For this review, take the finished solid that the model builds, in its own axes (mm). A direction names the side the tool comes from. Round coordinates to 2 decimals unless told otherwise and drop trailing zeros. Write each loop counter-clockwise with the first axis right and the second up, starting at its lowest first coordinate (ties: lowest second). Pieces come first, ordered by that corner, then holes. Notation, with made-up numbers: M -10.5,-6 L 12.5,-6 A17 ccw 12.5,19 Z; hole C 45,39 d1. An arc over 180 degrees is marked long. Answer in a Markdown table with one row per item.
```python
from build123d import *

# Parameters (mm, degrees)
SKETCH1_W               = 195
SKETCH1_H               = 20
BOSS_EXTRUDE1_DEPTH     = 4.9
SKETCH2_R               = 1.75
CUT_EXTRUDE1_DEPTH      = 6
CUT_EXTRUDE2_START      = -2
CUT_EXTRUDE2_DEPTH      = 4.25
SKETCH4_W               = 5.75
SKETCH4_H               = 4.25
CUT_EXTRUDE3_DEPTH      = 5.9
LPATTERN1_COUNT         = 3
LPATTERN1_PITCH         = 35
MIRROR1_COPY_1_SKETCH_R = 1.75
MIRROR1_COPY_1_DEPTH    = 6
MIRROR1_COPY_2_SKETCH_R = 1.75
MIRROR1_COPY_2_DEPTH    = 6
MIRROR1_START           = -2
MIRROR1_COPY_3_DEPTH    = 4.25
MIRROR1_COPY_4_DEPTH    = 4.25
MIRROR1_COPY_5_SKETCH_W = 5.75
MIRROR1_COPY_5_SKETCH_H = 4.25
MIRROR1_COPY_5_DEPTH    = 5.9
MIRROR1_COPY_6_SKETCH_W = 5.75
MIRROR1_COPY_6_SKETCH_H = 4.25
MIRROR1_COPY_6_DEPTH    = 5.9
SKETCH5_R               = 4.25
CUT_EXTRUDE4_DEPTH      = 6
CUT_EXTRUDE5_START      = -4.8
SKETCH6_R               = 2.625
CUT_EXTRUDE5_DEPTH      = 11.8
LPATTERN2_COUNT         = 2
LPATTERN2_PITCH         = 35
MIRROR2_COPY_1_SKETCH_R = 4.25
MIRROR2_COPY_1_DEPTH    = 6
MIRROR2_START           = -4.8
MIRROR2_COPY_2_SKETCH_R = 2.625
MIRROR2_COPY_2_DEPTH    = 11.8


with BuildPart() as part:
    # Sketch1 → Boss-Extrude1 (new body, symmetric)
    with BuildSketch(Plane.XY):
        Rectangle(SKETCH1_W, SKETCH1_H)
    extrude(amount=BOSS_EXTRUDE1_DEPTH, both=True)

    # Sketch2 → Cut-Extrude1 (cut)
    with BuildSketch(Plane(origin=(0, 10, 0), x_dir=(1, 0, 0), z_dir=(0, 1, 0))):
        with Locations((-87.5, 0)):
            Circle(SKETCH2_R)
    cut_extrude1 = extrude(amount=-CUT_EXTRUDE1_DEPTH, mode=Mode.SUBTRACT)

    # Sketch3 → Cut-Extrude2 (cut)
    with BuildSketch(Plane(origin=(0, 10, 0), x_dir=(1, 0, 0), z_dir=(0, 1, 0)).offset(CUT_EXTRUDE2_START)):
        Polygon((-87.5, 3.319764048), (-90.375, 1.659882024), (-90.375, -1.659882024), (-87.5, -3.319764048), (-84.625, -1.659882024), (-84.625, 1.659882024), align=None)
    cut_extrude2 = extrude(amount=-CUT_EXTRUDE2_DEPTH, mode=Mode.SUBTRACT)

    # Sketch4 → Cut-Extrude3 (cut, through all)
    with BuildSketch(Plane.XY):
        with Locations((-87.5, 5.875)):
            Rectangle(SKETCH4_W, SKETCH4_H)
    cut_extrude3 = extrude(amount=CUT_EXTRUDE3_DEPTH, mode=Mode.SUBTRACT)

    # LPattern1: Cut-Extrude1, Cut-Extrude2, Cut-Extrude3 ×3
    with Locations(*[(i * LPATTERN1_PITCH, 0, 0) for i in range(1, LPATTERN1_COUNT)]):
        add(cut_extrude1, mode=Mode.SUBTRACT)
        add(cut_extrude2, mode=Mode.SUBTRACT)
        add(cut_extrude3, mode=Mode.SUBTRACT)

    # Mirror1: Cut-Extrude1, Cut-Extrude2, Cut-Extrude3 across plane
    add(cut_extrude1.mirror(Plane(origin=(0, 0, 0), x_dir=(0, 0, 1), z_dir=(1, 0, 0))), mode=Mode.SUBTRACT)
    add(cut_extrude2.mirror(Plane(origin=(0, 0, 0), x_dir=(0, 0, 1), z_dir=(1, 0, 0))), mode=Mode.SUBTRACT)
    add(cut_extrude3.mirror(Plane(origin=(0, 0, 0), x_dir=(0, 0, 1), z_dir=(1, 0, 0))), mode=Mode.SUBTRACT)

    # Mirror1 copy 1 sketch → Mirror1 copy 1 (cut)
    with BuildSketch(Plane(origin=(-35, 10, 0), x_dir=(-1, 0, 0), z_dir=(0, 1, 0))):
        with Locations((-87.5, 0)):
            Circle(MIRROR1_COPY_1_SKETCH_R)
    extrude(amount=-MIRROR1_COPY_1_DEPTH, mode=Mode.SUBTRACT)

    # Mirror1 copy 2 sketch → Mirror1 copy 2 (cut)
    with BuildSketch(Plane(origin=(-70, 10, 0), x_dir=(-1, 0, 0), z_dir=(0, 1, 0))):
        with Locations((-87.5, 0)):
            Circle(MIRROR1_COPY_2_SKETCH_R)
    extrude(amount=-MIRROR1_COPY_2_DEPTH, mode=Mode.SUBTRACT)

    # Mirror1 copy 3 sketch → Mirror1 copy 3 (cut)
    with BuildSketch(Plane(origin=(-35, 10, 0), x_dir=(-1, 0, 0), z_dir=(0, 1, 0)).offset(MIRROR1_START)):
        Polygon((-87.5, -3.319764048), (-90.375, -1.659882024), (-90.375, 1.659882024), (-87.5, 3.319764048), (-84.625, 1.659882024), (-84.625, -1.659882024), align=None)
    extrude(amount=-MIRROR1_COPY_3_DEPTH, mode=Mode.SUBTRACT)

    # Mirror1 copy 4 sketch → Mirror1 copy 4 (cut)
    with BuildSketch(Plane(origin=(-70, 10, 0), x_dir=(-1, 0, 0), z_dir=(0, 1, 0)).offset(MIRROR1_START)):
        Polygon((-87.5, -3.319764048), (-90.375, -1.659882024), (-90.375, 1.659882024), (-87.5, 3.319764048), (-84.625, 1.659882024), (-84.625, -1.659882024), align=None)
    extrude(amount=-MIRROR1_COPY_4_DEPTH, mode=Mode.SUBTRACT)

    # Mirror1 copy 5 sketch → Mirror1 copy 5 (cut, through all)
    with BuildSketch(Plane(origin=(-35, 0, 0), x_dir=(-1, 0, 0), z_dir=(0, 0, 1))):
        with Locations((-87.5, -5.875)):
            Rectangle(MIRROR1_COPY_5_SKETCH_W, MIRROR1_COPY_5_SKETCH_H)
    extrude(amount=MIRROR1_COPY_5_DEPTH, mode=Mode.SUBTRACT)

    # Mirror1 copy 6 sketch → Mirror1 copy 6 (cut, through all)
    with BuildSketch(Plane(origin=(-70, 0, 0), x_dir=(-1, 0, 0), z_dir=(0, 0, 1))):
        with Locations((-87.5, -5.875)):
            Rectangle(MIRROR1_COPY_6_SKETCH_W, MIRROR1_COPY_6_SKETCH_H)
    extrude(amount=MIRROR1_COPY_6_DEPTH, mode=Mode.SUBTRACT)

    # Sketch5 → Cut-Extrude4 (cut)
    with BuildSketch(Plane.XY.offset(4.9)):
        with Locations((-70, 0)):
            Circle(SKETCH5_R)
    cut_extrude4 = extrude(amount=-CUT_EXTRUDE4_DEPTH, mode=Mode.SUBTRACT)

    # Sketch6 → Cut-Extrude5 (cut)
    with BuildSketch(Plane.XY.offset(-1.1).offset(CUT_EXTRUDE5_START)):
        with Locations((-70, 0)):
            Circle(SKETCH6_R)
    cut_extrude5 = extrude(amount=CUT_EXTRUDE5_DEPTH, mode=Mode.SUBTRACT)

    # LPattern2: Cut-Extrude4, Cut-Extrude5 ×2
    with Locations(*[(i * LPATTERN2_PITCH, 0, 0) for i in range(1, LPATTERN2_COUNT)]):
        add(cut_extrude4, mode=Mode.SUBTRACT)
        add(cut_extrude5, mode=Mode.SUBTRACT)

    # Mirror2: Cut-Extrude4, Cut-Extrude5 across plane
    add(cut_extrude4.mirror(Plane(origin=(0, 0, 0), x_dir=(0, 0, 1), z_dir=(1, 0, 0))), mode=Mode.SUBTRACT)
    add(cut_extrude5.mirror(Plane(origin=(0, 0, 0), x_dir=(0, 0, 1), z_dir=(1, 0, 0))), mode=Mode.SUBTRACT)

    # Mirror2 copy 1 sketch → Mirror2 copy 1 (cut)
    with BuildSketch(Plane(origin=(-35, 0, 4.9), x_dir=(-1, 0, 0), z_dir=(0, 0, 1))):
        with Locations((-70, 0)):
            Circle(MIRROR2_COPY_1_SKETCH_R)
    extrude(amount=-MIRROR2_COPY_1_DEPTH, mode=Mode.SUBTRACT)

    # Mirror2 copy 2 sketch → Mirror2 copy 2 (cut)
    with BuildSketch(Plane(origin=(-35, 0, -1.1), x_dir=(-1, 0, 0), z_dir=(0, 0, 1)).offset(MIRROR2_START)):
        with Locations((-70, 0)):
            Circle(MIRROR2_COPY_2_SKETCH_R)
    extrude(amount=MIRROR2_COPY_2_DEPTH, mode=Mode.SUBTRACT)


solid = part.part
```
Q1. Machinability: for faces 1 (the face through (18, 8, 2)), 2 (the face through (19.25, 9.01, 0.08)), 3 (the face through (-37.622, 0.115, -3.027)), which of the approach directions +Z, -Z, +X, -X, +Y, -Y give a long, thin tool a straight path to every point of the face, cutting with its end or side? Answer none if there is none.
Found:
| item | result |
|---|---|
| face 1 | +Z |
| face 2 | +Y |
| face 3 | +Z, -Z |
Q2. Take a section at A-A (x = 70). State the section outline as (y, z) points (3 decimals).
Found:
| item | result |
|---|---|
| outline | M -10,-4.9 L -2.625,-4.9 L -2.625,-1.1 L -4.25,-1.1 L -4.25,4.9 L -10,4.9 Z; M 2.625,-4.9 L 10,-4.9 L 10,4.9 L 4.25,4.9 L 4.25,-1.1 L 2.625,-1.1 Z |
Q3. Take a section at B-B (y = 0). State how many separate pieces and enclosed holes the cut face has, then the cut area to 3 significant figures.
Found:
| item | result |
|---|---|
| separate pieces | 5 |
| enclosed holes | 0 |
| area | 1,630 mm² |
Q4. For probe 1 along Z at (x, y) = (17.5, 8.75); probe 2 along Y at (x, z) = (54, 1); probe 3 along Y at (x, z) = (70, 0.3), list the stretches that pass through material, from the lowest coordinate up.
Found:
| item | result |
|---|---|
| probe 1 | -4.9 to -1.75, 1.75 to 4.9 |
| probe 2 | -10 to 3.75, 8 to 10 |
| probe 3 | -10 to -4.25, 4.25 to 10 |
Q5. Mouldability with a two-part tool opening along X and no side actions: class faces 4 (the face through (20.375, 6, 2)), 5 (the face through (85.831, 9.014, -0.526)), 6 (the face through (-1, 0, -4.9)) as +X half, -X half, draft (parallel to the pull), parting line (faces both ways), or undercut.
Found:
| item | result |
|---|---|
| face 4 | undercut |
| face 5 | undercut |
| face 6 | draft |
